Autodesk Inventor part; units mm, degrees
ref_plane "part_XY" through (0, 0, 0) normal (-1, 0, 0) x (0, 0, -1)
ref_plane "part_YZ" through (0, 0, 0) normal (0, 0, -1) x (0, -1, 0)
ref_plane "part_ZX" through (0, 0, 0) normal (0, -1, 0) x (-1, 0, 0)
sketch "Sketch_1" plane through (0, 0, 0) normal (0, 0, 1) x (1, 0, 0)
  line L0 (10, 0) -> (0, 0)
  line L1 (0, 3.5) -> (0.5, 3)
  line L2 (0.5, 3) -> (9.5, 3)
  line L3 (9.5, 3) -> (10, 3.5)
  line L4 (10, 3.5) -> (10, 10.5)
  line L5 (10, 10.5) -> (9.5, 11)
  line L6 (9.5, 11) -> (0.5, 11)
  line L7 (0.5, 11) -> (0, 10.5)
  line L8 (0, 10.5) -> (0, 3.5)
revolve "Revolution1" add sketch "Sketch_1" angle 360 about axis through (10, 0, 0) along (1, 0, 0)
sketch "Sketch_4" plane through (5, 0, 0) normal (1, 0, 0) x (0, 0, -1)
  line L0 (0, 1.5) -> (0, 11)
  line L1 (0, 11) -> (2, 11)
  line L2 (2, 11) -> (1.621, 10.621)
  line L3 (1.621, 10.621) -> (1.621, 1.5)
  line L4 (1.621, 1.5) -> (0, 1.5)
  line L5 (0, 1.5) -> (0, 11)
revolve "Revolution2" cut sketch "Sketch_4" angle 360 about axis through (5, 1.5, 0) along (0, -1, 0)
thread "Thread1"
sketch "Sketch_3" plane through (5, 0, 0) normal (1, 0, 0) x (0, 0, -1)
  line L0 (-1.5, 0) -> (-11, 0)
  line L1 (-11, 0) -> (-11, 2)
  line L2 (-11, 2) -> (-10.621, 1.621)
  line L3 (-10.621, 1.621) -> (-1.5, 1.621)
  line L4 (-1.5, 1.621) -> (-1.5, 0)
  line L5 (-1.5, 0) -> (-11, 0)
revolve "Revolution3" cut sketch "Sketch_3" angle 360 about axis through (5, 0, 1.5) along (0, 0, -1)
thread "Thread2"
sketch "Sketch_2" plane through (5, 0, 0) normal (1, 0, 0) x (0, 0, -1)
  line L0 (-1.25, 0) -> (-1.25, -4.2)
  line L1 (-1.25, -4.2) -> (1.25, -4.2)
  line L2 (1.25, -4.2) -> (1.25, 0)
  line L3 (1.25, 0) -> (-1.25, 0)
extrude "Extrusion1" cut sketch "Sketch_2" along normal mid plane 10
sketch "Sketch_6" plane through (5, 0, 0) normal (1, 0, 0) x (0, 0, -1)
  circle A0 centre (5.3033, 5.3033) radius 2.25
extrude "Extrusion2" cut sketch "Sketch_6" along normal mid plane 10
sketch "Sketch_7" plane through (5, 0, 0) normal (1, 0, 0) x (0, 0, -1)
  circle A0 centre (-5.3033, 5.3033) radius 2.25
extrude "Extrusion3" cut sketch "Sketch_7" along normal mid plane 10
sketch "Sketch_8" plane through (5, 0, 0) normal (1, 0, 0) x (0, 0, -1)
  circle A0 centre (-5.3033, -5.3033) radius 2.25
extrude "Extrusion4" cut sketch "Sketch_8" along normal mid plane 10
sketch "Sketch_9" plane through (5, 0, 0) normal (1, 0, 0) x (0, 0, -1)
  circle A0 centre (5.3033, -5.3033) radius 2.25
extrude "Extrusion5" cut sketch "Sketch_9" along normal mid plane 10
ref_plane "part_XY" through (0, 0, 0) normal (-1, 0, 0) x (0, 0, -1)
ref_plane "part_YZ" through (0, 0, 0) normal (0, 0, -1) x (0, -1, 0)
ref_plane "part_ZX" through (0, 0, 0) normal (0, -1, 0) x (-1, 0, 0)
properties part number "SC  0610CKP4"
The listing builds one solid part. Answer for the finished solid, in the listing's coordinates (mm). A direction names the side the tool comes from. Give positions to 0.01 mm unless a question says otherwise; leave off trailing zeros. Write each loop counter-clockwise with the first axis right and the second up, starting at its lowest first coordinate (ties: lowest second). Pieces come first, ordered by that corner, then holes.
Item 1: Which of the six approach directions +Z, -Z, +X, -X, +Y, -Y give full straight-line access (tool end or side, diameter ignored) to faces 5 (the flat face through (5, -4.2, 0)), 6 (the flat face through (0, 5, 0))?
Item 2: Determine the mould class of faces 1 (the conical face through (9.64, 3.14, -0.12)), 2 (the cylindrical face through (4.379, 1.497, 6.516)), 3 (the cylindrical face through (5.07, 7.534, 5.596)), 4 (the cylindrical face through (4.379, 6.516, -1.497)) for opening direction X: released by +X, released by -X, zero draft, split by the parting line, or undercut.
Item 3: Section C-C, the plane x = 1.25 is taken. Write down the section's boundary in (y, z), plus the area to 3 significant figures.
Item 4: Section B-B, the plane x = 5 is taken. Write down the section's boundary in (y, z).
Item 5: Find the intervals of material crossed by line 1 along X through (y, z) = (9, 0); line 2 along Y through (x, z) = (3.25, -4); line 3 along Z through (x, y) = (1.5, -3.25), in increasing order.
Item 6: Section A-A, the plane y = 0 is taken. Write down the section's boundary in (x, z), plus the area to 3 significant figures.
Item 7: Flat-ended cylindrical pins translate along their axes: P1, Ø1.6, axis at x = 3, y = -3.5, coming from the +Z side; P2, Ø1.9, axis at x = 5, z = 0, coming from the +Y side; P3, Ø0.7, axis at x = 5.5, y = -3.5, coming from the -Z side. Find the tip coordinate at first contact, or state that the pin passes through.
Item 8: Section D-D, the plane z = -6.75 is taken. Count the separate pieces of the cut face and the enclosed holes in it, plus the area to 3 significant figures.
Completed:
1. face 5: +X, -X
1. face 6: +Z, -Z, -X, +Y, -Y
2. face 1: released by +X
2. face 2: undercut
2. face 3: zero draft
2. face 4: undercut
3. outline: circle Ø22 at (0, 0); hole circle Ø4.5 at (-5.3, -5.3); hole circle Ø4.5 at (-5.3, 5.3); hole (-4.2, -1.25) - (-2.73, -1.25) arc R3 ccw (long way) to (-2.73, 1.25) - (-4.2, 1.25) - close; hole circle Ø4.5 at (5.3, -5.3); hole circle Ø4.5 at (5.3, 5.3)
3. area: 285 mm2
4. outline: (-4.2, -1.25) - (-4.2, 1.25) - (-2.73, 1.25) arc R3 cw to (-1.62, 2.52) - (-1.62, 10.62) - (-1.84, 10.84) arc R11 ccw (long way) to (10.84, -1.84) - (10.62, -1.62) - (2.52, -1.62) arc R3 cw to (-2.73, -1.25) - close; (1.62, 2.52) arc R3 cw to (2.52, 1.62) - (10.62, 1.62) - (10.84, 1.84) arc R11 ccw to (1.84, 10.84) - (1.62, 10.62) - close; hole circle Ø4.5 at (-5.3, -5.3); hole circle Ø4.5 at (-5.3, 5.3); hole circle Ø4.5 at (5.3, -5.3); hole circle Ø4.5 at (5.3, 5.3)
5. line 1: x = 0 to 3.38, 6.62 to 10
5. line 2: y = -10.25 to -7.14, -3.47 to 3.47, 7.14 to 10.25
5. line 3: z = -10.51 to -6.22, -4.38 to -1.25, 1.25 to 4.38, 6.22 to 10.51
6. outline: (0, -10.5) - (0.5, -11) - (9.5, -11) - (10, -10.5) - (10, -3.5) - (9.5, -3) - (0.5, -3) - (0, -3.5) - close; (0, 3.5) - (0.5, 3) - (3.38, 3) - (3.38, 10.62) - (3, 11) - (0.5, 11) - (0, 10.5) - close; (6.62, 3) - (9.5, 3) - (10, 3.5) - (10, 10.5) - (9.5, 11) - (7, 11) - (6.62, 10.62) - close
6. area: 133 mm2
7. P1: stops at z = 10.66
7. P2: stops at y = -4.2
7. P3: stops at z = -10.54
8. separate pieces: 3
8. enclosed holes: 0
8. area: 104 mm2
